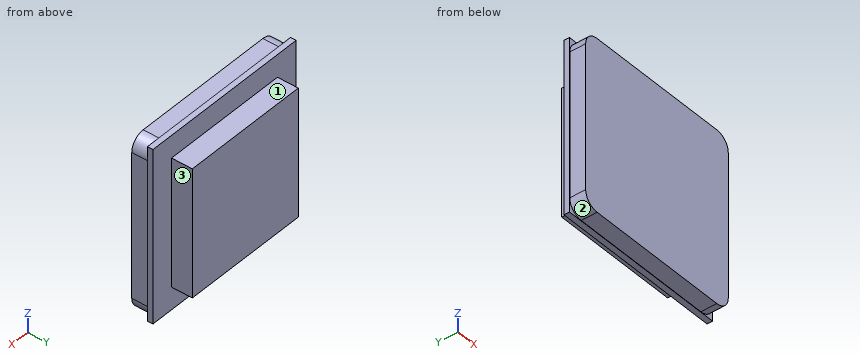
```python
from build123d import *

# Parameters (mm, degrees)
SKETCH1_W           = 25
SKETCH1_H           = 25
BOSS_EXTRUDE1_DEPTH = 0.8
SKETCH2_W           = 18.5
SKETCH2_H           = 18.5
BOSS_EXTRUDE2_DEPTH = 3
BOSS_EXTRUDE4_DEPTH = 2.3


with BuildPart() as part:
    # Sketch1 → Boss-Extrude1 (new body)
    with BuildSketch(Plane(origin=(0, 0, 0), x_dir=(1, 0, 0), z_dir=(0, 1, 0))):
        Rectangle(SKETCH1_W, SKETCH1_H)
    extrude(amount=BOSS_EXTRUDE1_DEPTH)

    # Sketch2 → Boss-Extrude2 (add)
    with BuildSketch(Plane(origin=(0, 0.8, 0), x_dir=(1, 0, 0), z_dir=(0, 1, 0))):
        Rectangle(SKETCH2_W, SKETCH2_H)
    extrude(amount=BOSS_EXTRUDE2_DEPTH)

    # Sketch3 → Boss-Extrude4 (add)
    with BuildSketch(Plane.XZ):
        with BuildLine():
            Line((-10.45, -12.45), (10.45, -12.45))
            ThreePointArc((10.45, -12.45), (11.864213562, -11.864213562), (12.45, -10.45))
            Line((12.45, -10.45), (12.45, 10.45))
            ThreePointArc((12.45, 10.45), (11.864213562, 11.864213562), (10.45, 12.45))
            Line((10.45, 12.45), (-10.45, 12.45))
            ThreePointArc((-10.45, 12.45), (-11.864213562, 11.864213562), (-12.45, 10.45))
            Line((-12.45, 10.45), (-12.45, -10.45))
            ThreePointArc((-12.45, -10.45), (-11.864213562, -11.864213562), (-10.45, -12.45))
        make_face()
    extrude(amount=BOSS_EXTRUDE4_DEPTH)


solid = part.part
```
The model under review builds one solid part; all positions refer to its coordinate system, in mm. Face numbers are marked on the shaded views. A direction names the side the tool comes from. Round coordinates to 2 decimals unless told otherwise and drop trailing zeros. Write each loop counter-clockwise with the first axis right and the second up, starting at its lowest first coordinate (ties: lowest second). Pieces come first, ordered by that corner, then holes. Notation, with made-up numbers: M -16,10 L 32,10 A26 cw 32,37 Z; hole C -18,42 d7. An arc over 180 degrees is marked long. Use CSV: the item, a comma, the result in double quotes. Start each with the question number.
(1) We need section B-B, the plane x = 5. State the section outline as (y, z) points.
(2) We need section A-A, the plane z = 6.25. State the section outline as (x, y) points, then the cut area to 3 significant figures.
(3) For line 1 along Y through (x, z) = (-10.5, -4.25); line 2 along X through (y, z) = (-1, -7); line 3 along Z through (x, y) = (-1.75, 1), list the stretches that pass through material, from the lowest coordinate up.
(4) We need section D-D, the plane x = -10.75. State the section outline as (y, z) points, then the cut area to 3 significant figures.
(5) Clearance check with flat-ended pins moving along their axes: P1, Ø1.2, axis at y = -1, z = -4, coming from the +X side; P2, Ø1.5, axis at x = 4, y = 3, coming from the -Z side; P3, Ø1.5, axis at y = 2, z = 1, coming from the +X side. State where each tip first meets the part, or that it passes through.
(6) Tool access review of the marked faces 1, 2 and 3: name each direction out of +Z, -Z, +X, -X, +Y, -Y from which nothing blocks a thin tool from reaching the whole face with its end or side.
(7) We need section C-C, the plane y = 1.75. State the section outline as (x, z) points, then the cut area to 3 significant figures.
Findings:
1,outline,"M -2.3,-12.45 L 0,-12.45 L 0,-12.5 L 0.8,-12.5 L 0.8,-9.25 L 3.8,-9.25 L 3.8,9.25 L 0.8,9.25 L 0.8,12.5 L 0,12.5 L 0,12.45 L -2.3,12.45 Z"
2,outline,"M -12.5,0 L -12.45,0 L -12.45,-2.3 L 12.45,-2.3 L 12.45,0 L 12.5,0 L 12.5,0.8 L 9.25,0.8 L 9.25,3.8 L -9.25,3.8 L -9.25,0.8 L -12.5,0.8 Z"
2,area,"133 mm^2"
3,line 1,"-2.3 to 0.8"
3,line 2,"-12.45 to 12.45"
3,line 3,"-9.25 to 9.25"
4,outline,"M -2.3,-12.43 L 0,-12.43 L 0,-12.5 L 0.8,-12.5 L 0.8,12.5 L 0,12.5 L 0,12.43 L -2.3,12.43 Z"
4,area,"77.2 mm^2"
5,P1,"x = 12.45"
5,P2,"z = -9.25"
5,P3,"x = 9.25"
6,face 1,"+Z, +X, -X, +Y"
6,face 2,"-Z, -X, -Y"
6,face 3,"+Z, -Z, +X, +Y"
7,outline,"M -9.25,-9.25 L 9.25,-9.25 L 9.25,9.25 L -9.25,9.25 Z"
7,area,"342 mm^2"
